```python
from build123d import *

# Parameters (mm, degrees)
SKETCH1_W           = 29.88
SKETCH1_H           = 35.71
SKETCH1_R           = 4
SKETCH1_R_2         = 0.75
BOSS_EXTRUDE1_DEPTH = 1.5
SKETCH2_R           = 0.94
BOSS_EXTRUDE2_DEPTH = 1.5
BOSS_EXTRUDE3_START = -1.5
SKETCH3_R           = 1
BOSS_EXTRUDE3_DEPTH = 1.5
FILLET1_R           = 0.75


with BuildPart() as part:
    # Sketch1 → Boss-Extrude1 (new body)
    with BuildSketch(Plane.XY):
        Rectangle(SKETCH1_W, SKETCH1_H)
        Circle(SKETCH1_R, mode=Mode.SUBTRACT)
        with Locations((4.772970773, 4.772970773)):
            Circle(SKETCH1_R_2, mode=Mode.SUBTRACT)
        with Locations(Location((4.772970773, -4.772970773, 0), (0, 0, 180))):
            Circle(SKETCH1_R_2, mode=Mode.SUBTRACT)
        with Locations((-4.772970773, -4.772970773)):
            Circle(SKETCH1_R_2, mode=Mode.SUBTRACT)
        with Locations(Location((-4.772970773, 4.772970773, 0), (0, 0, 180))):
            Circle(SKETCH1_R_2, mode=Mode.SUBTRACT)
    extrude(amount=BOSS_EXTRUDE1_DEPTH)

    # Sketch2 → Boss-Extrude2 (add)
    with BuildSketch(Plane(origin=(0, 17.855, 0), x_dir=(1, 0, 0), z_dir=(0, 1, 0))):
        Polygon((-14.94, 7.426000053), (-9.27, 7.426000053), (-9.27, 4.01933008), (9.27, 4.01933008), (9.27, 7.426000053), (12.62, 7.426000053), (14.94, 5.722665067), (14.94, -1.5), (-14.94, -1.5), align=None)
        with Locations(Location((-12.34, 3.986000053, 0), (0, 0, 270))):
            Circle(SKETCH2_R, mode=Mode.SUBTRACT)
        with BuildLine():
            ThreePointArc((12.66, 3.986000053), (11.66, 4.986000053), (10.66, 3.986000053))
            ThreePointArc((10.66, 3.986000053), (11.66, 2.986000053), (12.66, 3.986000053))
        make_face(mode=Mode.SUBTRACT)
    extrude(amount=-BOSS_EXTRUDE2_DEPTH)

    # Sketch3 → Boss-Extrude3 (add)
    with BuildSketch(Plane.XZ.offset(17.855).offset(BOSS_EXTRUDE3_START)):
        Polygon((-14.94, 1.5), (14.94, 1.5), (14.94, -5.722665067), (12.62, -7.426000053), (9.27, -7.426000053), (9.27, -4.01933008), (-5.44, -4.01933008), (-5.44, -7.426000053), (-14.94, -7.426000053), align=None)
        with Locations(Location((11.66, -3.986000053, 0), (0, 0, 90))):
            Circle(SKETCH3_R, mode=Mode.SUBTRACT)
        with Locations(Location((-8.34, -3.986000053, 0), (0, 0, 270))):
            Circle(SKETCH3_R, mode=Mode.SUBTRACT)
    extrude(amount=BOSS_EXTRUDE3_DEPTH)

    # Fillet1
    fillet1_edges = [part.edges().sort_by_distance(p)[0] for p in [
        (0, -17.855, 1.5),
        (-14.94, 17.105, -7.426000053),
        (-9.27, 17.105, -7.426000053),
        (-9.27, 17.105, -4.01933008),
        (9.27, 17.105, -4.01933008),
        (9.27, 17.105, -7.426000053),
        (12.62, 17.105, -7.426000053),
        (14.94, 17.105, -5.722665067),
        (0, 16.355, 0),
        (0, 17.855, 1.5),
        (0, -16.355, 0),
        (-14.94, -17.105, -7.426000053),
        (14.94, -17.105, -5.722665067),
        (12.62, -17.105, -7.426000053),
        (9.27, -17.105, -7.426000053),
        (9.27, -17.105, -4.01933008),
        (-5.44, -17.105, -4.01933008),
        (-5.44, -17.105, -7.426000053),
    ]]
    fillet(fillet1_edges, radius=FILLET1_R)


solid = part.part
```
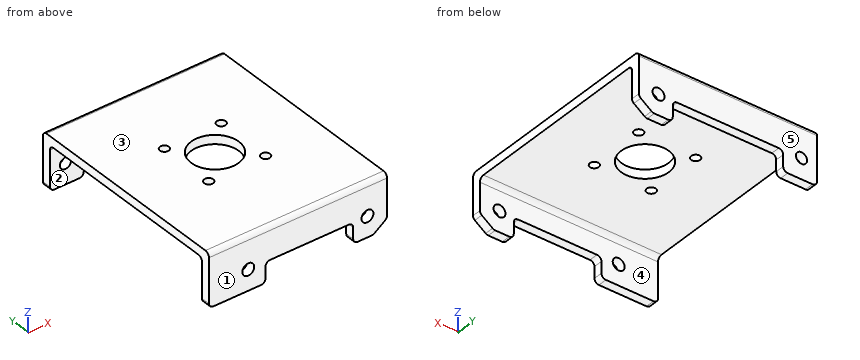
The listing builds one solid part. Answer for the finished solid, in the listing's coordinates (mm). Face numbers are marked on the shaded views. A direction names the side the tool comes from. Coordinates: 2 decimals unless noted, no trailing zeros. Loops run counter-clockwise (first coordinate to the right, second up) from the corner with the lowest first, then second, coordinate; pieces in that order, holes last. Notation, with made-up numbers: (89, -14.75) - (127, -14.75) arc R23 ccw to (127, -4.75) - close; hole circle Ø6 at (42, 0). An arc over 180 degrees is marked (long way). Write item = value, one per line.
1) Section C-C (y = 0) is taken. Determine the outline of the cut face in (x, z).
Responses:
outline = (-14.94, 0) - (-4, 0) - (-4, 1.5) - (-14.94, 1.5) - close; (4, 0) - (14.94, 0) - (14.94, 1.5) - (4, 1.5) - close
2) Find the intervals of material crossed by line 1 along Y through (x, z) = (-12.5, -2) (3 decimals); line 2 along Z through (x, y) = (11.66, 16.95); line 3 along Z through (x, y) = (-10, 15), in increasing order.
Responses:
line_1 = -17.855 to -16.355, 16.355 to 17.855
line_2 = -7.43 to -4.99, -2.99 to 1.5
line_3 = 0 to 1.5
3) Determine the mould class of the marked faces 3, 4 and 5 for opening direction Y: pulls with the +Y half, pulls with the -Y half, needs draft (parallel to the pull), parting line crosses it, or undercut.
Responses:
face_3 = needs draft
face_4 = undercut
face_5 = pulls with the +Y half
4) Each of these flat-tipped pins is pushed along its axis until it touches: P1, Ø9, axis at x = -7, y = 3.5, coming from the -Z side; P2, Ø1.6, axis at x = 2, y = 17, coming from the -Z side; P3, Ø1.7, axis at x = -12.34, z = -3.986, coming from the +Y side (3 decimals). Where does it stop, or does it pass through?
Responses:
P1 = 0
P2 = -4.02
P3 = -16.355
5) Section B-B (x = 0) is taken. Determine the outline of the cut face in (y, z) (3 decimals).
Responses:
outline = (-17.855, -4.019) - (-16.355, -4.019) - (-16.355, -0.75) arc R0.75 cw to (-15.605, 0) - (-4, 0) - (-4, 1.5) - (-17.105, 1.5) arc R0.75 ccw to (-17.855, 0.75) - close; (4, 0) - (15.605, 0) arc R0.75 cw to (16.355, -0.75) - (16.355, -4.019) - (17.855, -4.019) - (17.855, 0.75) arc R0.75 ccw to (17.105, 1.5) - (4, 1.5) - close
6) Section A-A (z = -1.25) is taken. Determine the outline of the cut face in (x, y) (3 decimals), plus the area to 3 significant figures.
Responses:
outline = (-14.94, -17.855) - (14.94, -17.855) - (14.94, -16.355) - (-14.94, -16.355) - close; (-14.94, 16.355) - (14.94, 16.355) - (14.94, 17.855) - (-14.94, 17.855) - close
area = 89.6 mm^2
7) Which of the six approach directions +Z, -Z, +X, -X, +Y, -Y give full straight-line access (tool end or side, diameter ignored) to the marked faces 1 and 2?
Responses:
face_1 = +Z, -Z, +X, -X, -Y
face_2 = -Z, +X, -X
8) Section D-D (x = 7) is taken. Determine the outline of the cut face in (y, z) (3 decimals).
Responses:
outline = (-17.855, -4.019) - (-16.355, -4.019) - (-16.355, -0.75) arc R0.75 cw to (-15.605, 0) - (15.605, 0) arc R0.75 cw to (16.355, -0.75) - (16.355, -4.019) - (17.855, -4.019) - (17.855, 0.75) arc R0.75 ccw to (17.105, 1.5) - (-17.105, 1.5) arc R0.75 ccw to (-17.855, 0.75) - close
